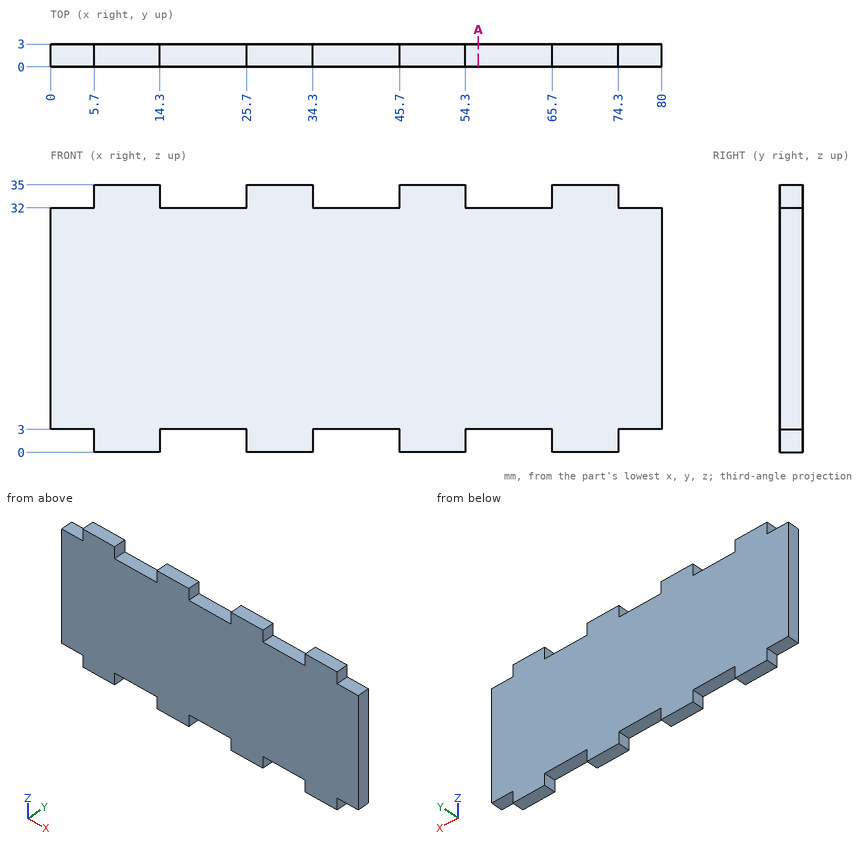
Check sheet for the drawn part. Datum: minimum x, y, z corner. Units: mm. Round coordinates to 2 decimals unless told otherwise and drop trailing zeros. Write each loop counter-clockwise with the first axis right and the second up, starting at its lowest first coordinate (ties: lowest second). Pieces come first, ordered by that corner, then holes. Notation, with made-up numbers: (53, 79.5) - (95, 79.5) arc R30 ccw to (95, 106.5) - close; hole circle Ø9 at (-35.5, 15.5). An arc over 180 degrees is marked (long way). Return JSON: item names as keys, results as strings.
Q1. Scan lines: L1, parallel to X at y = 1.05, z = 33.5; L2, parallel to Z at x = 58, y = 0.45. Record each from-to range of solid material in increasing order. Write a range as from..to.
Returned:
{"L1": "x = 5.7..14.3, 25.7..34.3, 45.7..54.3, 65.7..74.3", "L2": "z = 3..32"}
Q2. Depth check by flat-ended pin: P1, Ø0.9, axis at x = 60.5, y = 1, coming from the +Z side; P2, Ø0.9, axis at y = 1.5, z = 1.5, coming from the +X side; P3, Ø1.5, axis at y = 2, z = 2, coming from the -X side. Enter the tip coordinate at first touch or a pass-through.
Returned:
{"P1": "stops at z = 32", "P2": "stops at x = 74.3", "P3": "stops at x = 5.7"}
Q3. Cross-section at A-A (x = 56). Record the boundary of the cut face in (y, z).
Returned:
{"outline": "(0, 3) - (3, 3) - (3, 32) - (0, 32) - close"}
